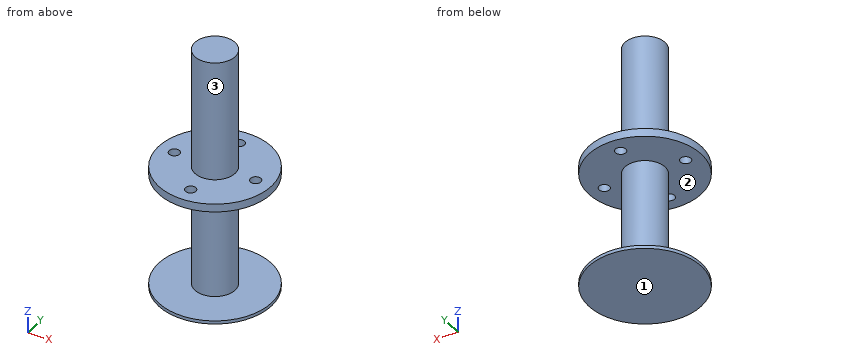
from build123d import *

# Parameters (mm, degrees)
SKETCH1_R                = 70
SKETCH1_R_2              = 6.5
BOSS_EXTRUDE1_DEPTH      = 10
SKETCH2_R                = 25
BOSS_EXTRUDE2_DEPTH      = 150
BOSS_EXTRUDE2_DEPTH_BACK = 150
SKETCH3_R                = 70
BOSS_EXTRUDE3_DEPTH      = 4


with BuildPart() as part:
    # Sketch1 → Boss-Extrude1 (new body)
    with BuildSketch(Plane.XY):
        Circle(SKETCH1_R)
        with Locations((0, 50)):
            Circle(SKETCH1_R_2, mode=Mode.SUBTRACT)
        with Locations((50, 0)):
            Circle(SKETCH1_R_2, mode=Mode.SUBTRACT)
        with Locations((0, -50)):
            Circle(SKETCH1_R_2, mode=Mode.SUBTRACT)
        with Locations((-50, 0)):
            Circle(SKETCH1_R_2, mode=Mode.SUBTRACT)
    extrude(amount=BOSS_EXTRUDE1_DEPTH)

    # Sketch2 → Boss-Extrude2 (add, two sides)
    with BuildSketch(Plane.XY.offset(10)) as boss_extrude2_sk:
        Circle(SKETCH2_R)
    extrude(amount=BOSS_EXTRUDE2_DEPTH)
    extrude(boss_extrude2_sk.sketch, amount=-BOSS_EXTRUDE2_DEPTH_BACK)

    # Sketch3 → Boss-Extrude3 (add)
    with BuildSketch(Plane(origin=(0, 0, -140), x_dir=(-1, 0, 0), z_dir=(0, 0, -1))):
        Circle(SKETCH3_R)
    extrude(amount=BOSS_EXTRUDE3_DEPTH)


solid = part.part
The listing builds one solid part. Answer for the finished solid, in the listing's coordinates (mm). Face numbers are marked on the shaded views. A direction names the side the tool comes from. Give positions to 0.01 mm unless a question says otherwise; leave off trailing zeros. Write each loop counter-clockwise with the first axis right and the second up, starting at its lowest first coordinate (ties: lowest second). Pieces come first, ordered by that corner, then holes.
Item 1: Section B-B, the plane x = -38 is taken. Write down the section's boundary in (y, z).
Item 2: Find the intervals of material crossed by line 1 along Y through (x, z) = (0, 2.5); line 2 along Z through (x, y) = (50, 11); line 3 along Y through (x, z) = (50, 5), in increasing order.
Item 3: Section C-C, the plane y = -31.5 is taken. Write down the section's boundary in (x, z).
Item 4: Section D-D, the plane x = 50 is taken. Write down the section's boundary in (y, z), plus the area to 3 significant figures.
Item 5: Section A-A, the plane y = 0 is taken. Write down the section's boundary in (x, z), plus the area to 3 significant figures.
Item 6: Which of the six approach directions +Z, -Z, +X, -X, +Y, -Y give full straight-line access (tool end or side, diameter ignored) to the marked faces 1, 2 and 3?
Item 7: Flat-ended cylindrical pins translate along their axes: P1, Ø3, axis at x = -33, z = 12.5, coming from the -Y side; P2, Ø1, axis at x = -6, z = 116, coming from the +Y side; P3, Ø17, axis at x = 0, y = 50, coming from the +Z side; P4, Ø11.5, axis at x = -50, y = 0, coming from the +Z side. Find the tip coordinate at first contact, or state that the pin passes through.
Completed:
1. outline: (-58.79, -144) - (58.79, -144) - (58.79, -140) - (-58.79, -140) - close; (-58.79, 0) - (58.79, 0) - (58.79, 10) - (-58.79, 10) - close
2. line 1: y = -70 to -56.5, -43.5 to 43.5, 56.5 to 70
2. line 2: z = -144 to -140, 0 to 10
2. line 3: y = -48.99 to -6.5, 6.5 to 48.99
3. outline: (-62.51, -144) - (62.51, -144) - (62.51, -140) - (-62.51, -140) - close; (-62.51, 0) - (62.51, 0) - (62.51, 10) - (-62.51, 10) - close
4. outline: (-48.99, -144) - (48.99, -144) - (48.99, -140) - (-48.99, -140) - close; (-48.99, 0) - (-6.5, 0) - (-6.5, 10) - (-48.99, 10) - close; (6.5, 0) - (48.99, 0) - (48.99, 10) - (6.5, 10) - close
4. area: 1,240 mm2
5. outline: (-70, -144) - (70, -144) - (70, -140) - (25, -140) - (25, 0) - (43.5, 0) - (43.5, 10) - (25, 10) - (25, 160) - (-25, 160) - (-25, 10) - (-43.5, 10) - (-43.5, 0) - (-25, 0) - (-25, -140) - (-70, -140) - close; (-70, 0) - (-56.5, 0) - (-56.5, 10) - (-70, 10) - close; (56.5, 0) - (70, 0) - (70, 10) - (56.5, 10) - close
5. area: 16,200 mm2
6. face 1: -Z, +X, -X, +Y, -Y
6. face 2: none
6. face 3: +Z
7. P1: passes through
7. P2: stops at y = 24.39
7. P3: stops at z = 10
7. P4: stops at z = -140
